```python
from build123d import *

# Parameters (mm, degrees)
SKETCH1_W           = 200
SKETCH1_H           = 80
BOSS_EXTRUDE1_DEPTH = 35
SKETCH2_W           = 5
SKETCH2_H           = 6
CUT_EXTRUDE1_DEPTH  = 201
CUT_EXTRUDE5_DEPTH  = 201


with BuildPart() as part:
    # Sketch1 → Boss-Extrude1 (new body)
    with BuildSketch(Plane(origin=(0, 0, 0), x_dir=(1, 0, 0), z_dir=(0, 1, 0))):
        Rectangle(SKETCH1_W, SKETCH1_H)
    extrude(amount=BOSS_EXTRUDE1_DEPTH)

    # Sketch2 → Cut-Extrude1 (cut, through all)
    with BuildSketch(Plane.ZY.offset(100)):
        with Locations((37.5, 3)):
            Rectangle(SKETCH2_W, SKETCH2_H)
    extrude(amount=-CUT_EXTRUDE1_DEPTH, mode=Mode.SUBTRACT)

    # Sketch6 → Cut-Extrude5 (cut, through all)
    with BuildSketch(Plane(origin=(100, 0, 0), x_dir=(0, 0, -1), z_dir=(1, 0, 0))):
        Polygon((40, 22), (40, 23), (39, 22), (40, 21), align=None)
    extrude(amount=-CUT_EXTRUDE5_DEPTH, mode=Mode.SUBTRACT)


solid = part.part
```
Input: part model. Units: mm. Frame: model coordinates. A direction names the side the tool comes from. Round coordinates to 2 decimals unless told otherwise and drop trailing zeros.
1) Material intervals for line 1 (Z direction, x = -41.5, y = 2), sorted ascending.
Ans:
line 1: z = -40 to 35
2) Pin query (flat end, axial travel): pin 1 (6 mm diameter, centred on x = 73, z = 26, fed in from -Y); pin 2 (1.8 mm diameter, centred on x = -42.5, y = 4, fed in from +Z); pin 3 (1.5 mm diameter, centred on x = -15, z = 37.5, fed in from -Y). Return the tip coordinate at first contact, or that it passes through.
Ans:
pin 1: stops at y = 0
pin 2: stops at z = 35
pin 3: stops at y = 6
3) Set-up query: faces 1 (the flat face through (-100, 17, 1)), 2 (the flat face through (-1, 3, 35)). Return all of +Z, -Z, +X, -X, +Y, -Y with unobstructed straight access to the full face (end or side cutting, diameter ignored); none if empty.
Ans:
face 1: +Z, -Z, -X, +Y, -Y
face 2: +Z, +X, -X, -Y
